Autodesk Inventor part; units mm, degrees
ref_plane "Work Plane1" through (2.75, 0, 0) normal (0, -1, 0) x (1, 0, 0)
ref_plane "YZ Plane" through (0, 0, 0) normal (1, 0, 0) x (0, 1, 0)
ref_plane "XZ Plane" through (0, 0, 0) normal (0, 1, 0) x (-1, 0, 0)
sketch "Schizzo1" plane through (0, 0, 0) normal (0, 0, 1) x (1, 0, 0)
  line L0 (20, 3) -> (20, 0)
  line L1 (-20, 0) -> (20, 0)
  line L2 (-28, 0) -> (28, 0)
  line L3 (0, 3.6) -> (0, -0.6)
  line L4 (-20, 3) -> (-20, 0)
  line L5 (0, 3) -> (0, 0) construction
  line L6 (-28, 0) -> (28, 0)
  line L7 (-20, 3) -> (20, 3)
  dimension "d13" = 6
  dimension "d87" = 40
  dimension "d88" = 20
revolve "Corpo" add sketch "Schizzo1" angle 360 about axis through (-20, 0, 0) along (1, 0, 0)
thread "Filettatura1"
chamfer "Smusso1" distance 0.702 angle 45 1 edges at (20, -3, 0) measured on face at (6.6667, 2.9612, -0.4812)
chamfer "Smusso2" distance 0.702 angle 45 1 edges at (-20, -3, 0) measured on face at (6.1987, 2.9903, -0.2414)
ref_plane "Work Plane1" through (2.75, 0, 0) normal (0, -1, 0) x (1, 0, 0)
equation "\"d13\" = NND"
equation "\"d87\" = NLG"
equation "\"d88\" = 0.5 * NLG"
equation "\"d1\" = GEL"
equation "\"d9\" = -0.5 * SPD + 0.5 * NND"
equation "\"d10\" = -0.5 * SPD + 0.5 * NND"
equation "\"d11\" = -0.5 * SPD + 0.5 * NND"
equation "\"d12\" = -0.5 * SPD + 0.5 * NND"
equation "\"NLG\" = 40"
equation "\"GEL\" = NLG"
equation "\"GAL\" = 0.61345 * PTC"
equation "\"SPD\" = 4.596"
equation "\"d0\" = NND"
equation "\"GUL\" = 0.61345 * PTC"
equation "\"NND\" = 6"
equation "\"GUL1\" = GUL"
equation "\"GAL1\" = GAL"
equation "\"d80\" = -GUL - GEL"
equation "\"d86\" = -GEL + GUL1"
equation "\"PTC\" = 1"
equation "\"THREADDIA\" = 6"
equation "\"TOA\" = 30deg"
equation "\"GD1\" = THREADDIA - 1.2269 * PTC"
properties part number "DIN 976-1 - M6 x 40 - B" material "Acciaio, Dolce"
For this review, take the finished solid that the model builds, in its own axes (mm). Give positions to 0.01 mm unless a question says otherwise; leave off trailing zeros. Write each loop counter-clockwise with the first axis right and the second up, starting at its lowest first coordinate (ties: lowest second). Pieces come first, ordered by that corner, then holes.
Item 1: Wall thickness on probe 1 along Y at (x, z) = (-14.5, -0.15); probe 2 along Y at (x, z) = (0.5, -1); probe 3 along Z at (x, y) = (7.5, 2.75): over which ranges is each line inside the solid? List them lowest first.
Item 2: Take a section at A-A (x = 7). Give the boundary of the cut face in (y, z).
Item 3: Insertion check: P1, Ø2, axis at x = 6, z = 1.5, coming from the +Y side; P2, Ø1, axis at x = -6.5, y = 2, coming from the -Z side. Each pin has a flat end and moves straight along its axis. Give the tip position at first contact, or say it passes through.
Established:
1. probe 1: y = -3 to 3
1. probe 2: y = -2.83 to 2.83
1. probe 3: z = -1.2 to 1.2
2. outline: circle Ø6 at (0, 0)
3. P1: stops at y = 2.96
3. P2: stops at z = -2.6
